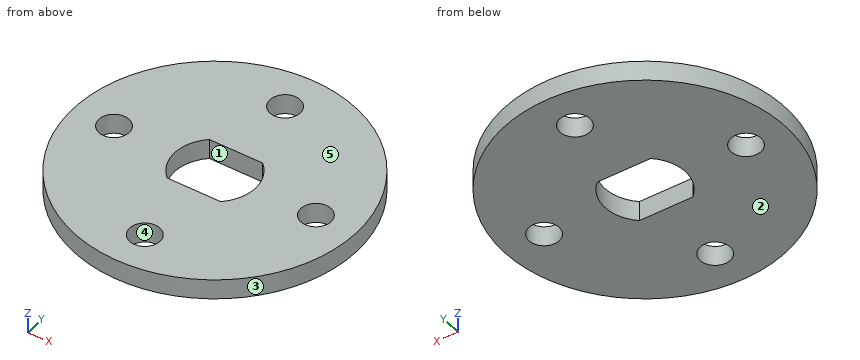
```python
from build123d import *

# Parameters (mm, degrees)
SKETCH_1_R          = 14
SKETCH_1_R_2        = 1.5
EXTRUDE_1_DEPTH     = 2
CUT_EXTRUDE_1_DEPTH = 20.899748742


with BuildPart() as part:
    # 草图1 → 凸台-拉伸1 (new body)
    with BuildSketch(Plane.XY):
        Circle(SKETCH_1_R)
        with Locations((0, 10)):
            Circle(SKETCH_1_R_2, mode=Mode.SUBTRACT)
        with Locations((10, 0)):
            Circle(SKETCH_1_R_2, mode=Mode.SUBTRACT)
        with Locations((-10, 0)):
            Circle(SKETCH_1_R_2, mode=Mode.SUBTRACT)
        with Locations((0, -10)):
            Circle(SKETCH_1_R_2, mode=Mode.SUBTRACT)
    extrude(amount=EXTRUDE_1_DEPTH)

    # 草图2 → 切除-拉伸1 (cut, through all)
    with BuildSketch(Plane(origin=(0, 0, 0), x_dir=(-1, 0, 0), z_dir=(0, 0, -1))):
        with BuildLine():
            ThreePointArc((-2.645751311, 3), (-4, 0), (-2.645751311, -3))
            Line((-2.645751311, -3), (2.645751311, -3))
            ThreePointArc((2.645751311, -3), (4, 0), (2.645751311, 3))
            Line((2.645751311, 3), (-2.645751311, 3))
        make_face()
    extrude(amount=-CUT_EXTRUDE_1_DEPTH, mode=Mode.SUBTRACT)


solid = part.part
```
Can you work these out from the model? Positions are in its coordinate system, mm. Face numbers are marked on the shaded views. A direction names the side the tool comes from. Coordinates: 2 decimals unless noted, no trailing zeros. Loops run counter-clockwise (first coordinate to the right, second up) from the corner with the lowest first, then second, coordinate; pieces in that order, holes last. Notation, with made-up numbers: (67.5, 14) - (101.5, 14) arc R15 cw to (101.5, 27) - close; hole circle Ø5 at (59, -6.5). An arc over 180 degrees is marked (long way). Answer as CSV lines item,"result". Start each with the question number.
1) Thinking about a two-plate mould opening in X: for the marked faces 3, 4 and 5, which applies, pulls with the +X half, pulls with the -X half, needs draft (parallel to the pull), parting line crosses it, or undercut?
2) I need wall thicknesses on line 1 (Y direction, x = 0, z = 1.5); line 2 (X direction, y = -11.25, z = 0.5); line 3 (Y direction, x = 9, z = 1.2). Which ranges of each line are inside material? Lowest first, please. Write a range as from..to.
3) Suppose I cut it at A-A (z = 1.6). Please give me the cut outline in (x, y), plus the area to 3 significant figures.
4) For pin 1 (4 mm diameter, centred on x = 0, y = -10, fed in from -Z); pin 2 (2.5 mm diameter, centred on x = 0, y = 10, fed in from +Z), each with a flat end and sliding along its axis, tell me the tip position at first contact or that it passes through.
5) Suppose I cut it at C-C (y = 10). Please give me the cut outline in (x, z), plus the area to 3 significant figures.
6) Which directions (+Z, -Z, +X, -X, +Y, -Y) give clear straight access to the entire face, cutting with the end or side of a thin tool? Please do the marked faces 1 and 2.
7) Suppose I cut it at B-B (x = 0). Please give me the cut outline in (y, z), plus the area to 3 significant figures.
Check result:
1,face 3,"parting line crosses it"
1,face 4,"undercut"
1,face 5,"needs draft"
2,line 1,"y = -14..-11.5, -8.5..-3, 3..8.5, 11.5..14"
2,line 2,"x = -8.33..-0.83, 0.83..8.33"
2,line 3,"y = -10.72..-1.12, 1.12..10.72"
3,outline,"circle Ø28 at (0, 0); hole circle Ø3 at (-10, 0); hole (-2.65, -3) - (2.65, -3) arc R4 ccw to (2.65, 3) - (-2.65, 3) arc R4 ccw to start; hole circle Ø3 at (0, -10); hole circle Ø3 at (0, 10); hole circle Ø3 at (10, 0)"
3,area,"544 mm²"
4,pin 1,"stops at z = 0"
4,pin 2,"passes through"
5,outline,"(-9.8, 0) - (-1.5, 0) - (-1.5, 2) - (-9.8, 2) - close; (1.5, 0) - (9.8, 0) - (9.8, 2) - (1.5, 2) - close"
5,area,"33.2 mm²"
6,face 1,"+Z, -Z"
6,face 2,"-Z, +X, -X, +Y, -Y"
7,outline,"(-14, 0) - (-11.5, 0) - (-11.5, 2) - (-14, 2) - close; (-8.5, 0) - (-3, 0) - (-3, 2) - (-8.5, 2) - close; (3, 0) - (8.5, 0) - (8.5, 2) - (3, 2) - close; (11.5, 0) - (14, 0) - (14, 2) - (11.5, 2) - close"
7,area,"32.0 mm²"
